Can you work these out from the drawing? Everything is in mm from the part's minimum corner. A direction names the side the tool comes from. Round coordinates to 2 decimals unless told otherwise and drop trailing zeros. Order: outer loops, then holes, each group sorted by start corner. A loop starts at its lowest first (then second) coordinate and runs counter-clockwise, first axis right, second up. Notation, with made-up numbers: M -36.5,12.25 L 13.5,12.25 A25 ccw 13.5,38.25 Z; hole C 33.25,11 d2. An arc over 180 degrees is marked long. Answer as a JSON object with one key per item and string values. Group by question number.
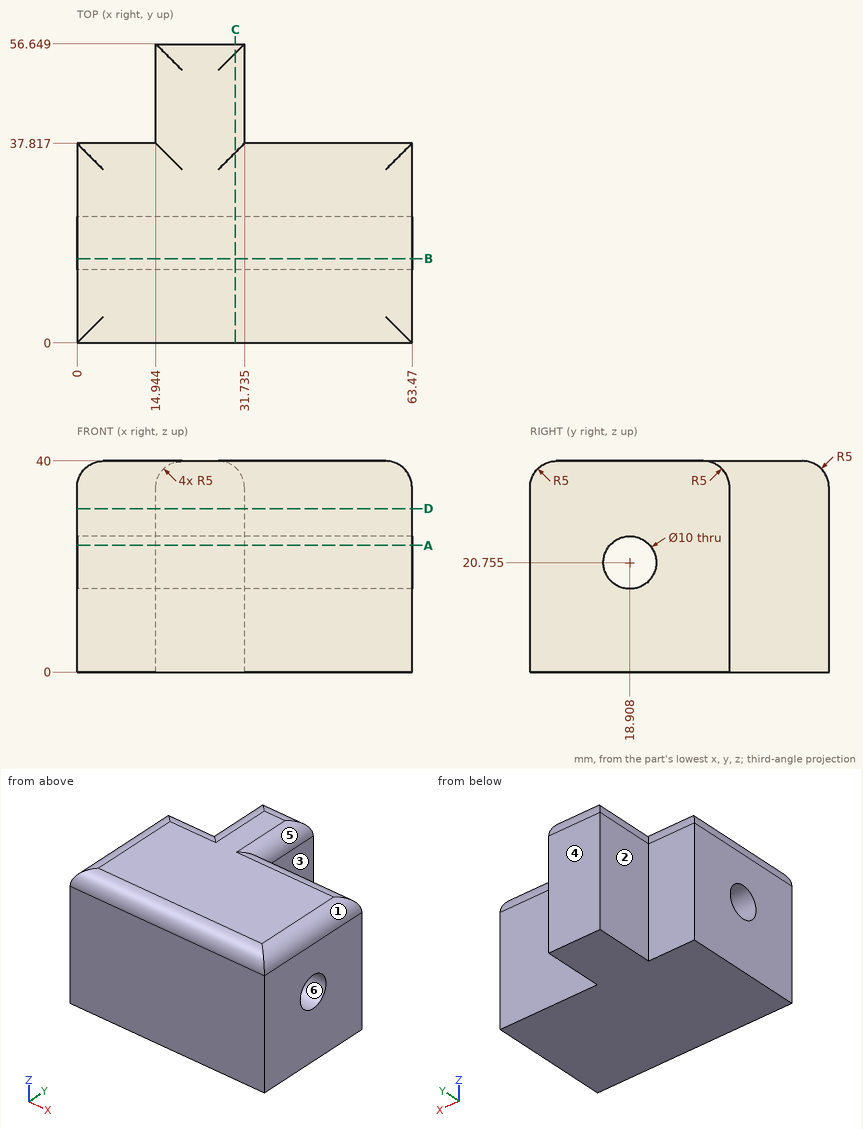
Item 1: If we mould it in two halves opening along Z, with no side actions, what happens to the marked faces 4, 5 and 6? For each: +Z half, -Z half, draft (parallel to the pull), parting line (faces both ways), or undercut.
Item 2: On a 3-axis mill with a long thin cutter (end or side, diameter ignored), from which of +Z, -Z, +X, -X, +Y, -Y can I reach the whole of each face in a straight line? I mean the marked faces 1, 2 and 3. Say none if no direction works.
Item 3: Suppose I cut it at B-B, the plane y = 16. Write out the boundary of the cut face in (x, z), and give its area (3 significant figures).
Item 4: Suppose I cut it at A-A, the plane z = 24. Write out the boundary of the cut face in (x, y) (1 decimal), and give its area (3 significant figures).
Item 5: Suppose I cut it at C-C, the plane x = 30. Write out the boundary of the cut face in (y, z) (1 decimal), and give its area (3 significant figures).
Item 6: I need wall thicknesses on line 1 (X direction, y = 45.5, z = 32) (1 decimal); line 2 (Y direction, x = 41.5, z = 34.5); line 3 (Z direction, x = 35.5, y = 23.5) (1 decimal). Which ranges of each line are inside material? Lowest first, please.
Item 7: I'm going to push flat-ended pins straight in: pin 1 Ø20.5 at (y, z) = (51.5, 15.5) entering from -X (1 decimal); pin 2 Ø1.5 at (x, z) = (42, 33.5) entering from +Y; pin 3 Ø15 at (y, z) = (50, 9) entering from +X (1 decimal). Where does each tip first touch, or does it pass through?
Item 8: Suppose I cut it at D-D, the plane z = 31. Write out the boundary of the cut face in (x, y) (1 decimal), and give its area (3 significant figures).
Computed:
{
 "1": {"face 4": "draft", "face 5": "+Z half", "face 6": "undercut"},
 "2": {"face 1": "+Z, +X, +Y, -Y", "face 2": "+Z, -Z, -X, +Y", "face 3": "+Z, -Z, +X, +Y"},
 "3": {"outline": "M 0,0 L 63.47,0 L 63.47,16.69 L 0,16.69 Z; M 0,24.82 L 63.47,24.82 L 63.47,35 A5 ccw 58.47,40 L 5,40 A5 ccw 0,35 Z", "area": "2,010 mm^2"},
 "4": {"outline": "M 0,0 L 63.5,0 L 63.5,15.1 L 0,15.1 Z; M 0,22.7 L 63.5,22.7 L 63.5,37.8 L 31.7,37.8 L 31.7,56.6 L 14.9,56.6 L 14.9,37.8 L 0,37.8 Z", "area": "2,230 mm^2"},
 "5": {"outline": "M 0,0 L 56.6,0 L 56.6,35 A5 ccw 54.9,38.8 L 36.1,38.8 A5 ccw 32.8,40 L 5,40 A5 ccw 0,35 Z; hole C 18.9,20.8 d10", "area": "2,150 mm^2"},
 "6": {"line 1": "x = 14.9 to 31.7", "line 2": "y = 0 to 37.82", "line 3": "z = 0 to 18.8, 22.7 to 40"},
 "7": {"pin 1": "stops at x = 14.9", "pin 2": "stops at y = 37.82", "pin 3": "stops at x = 31.7"},
 "8": {"outline": "M 0,0 L 63.5,0 L 63.5,37.8 L 31.7,37.8 L 31.7,56.6 L 14.9,56.6 L 14.9,37.8 L 0,37.8 Z", "area": "2,720 mm^2"}
}
